Design review of the part built by this model. Coordinates are the model's own, in mm. Round coordinates to 2 decimals unless told otherwise and drop trailing zeros. Loops run counter-clockwise (first coordinate to the right, second up) from the corner with the lowest first, then second, coordinate; pieces in that order, holes last. Notation, with made-up numbers: (82, 11.25) - (88, 11.25) arc R22 ccw to (88, 30.25) - close; hole circle Ø11 at (-7, 57). An arc over 180 degrees is marked (long way). Return JSON: item names as keys, results as strings. Group by question number.
(1) We need section C-C, the plane x = -12.7. Write out the cut boundary in (y, z).
(2) We need section A-A, the plane y = -19.05. Write out the cut boundary in (x, z) (3 decimals).
(3) We need section B-B, the plane x = 0. Write out the cut boundary in (y, z), and give its area (3 significant figures).
(4) Wall thickness on L1, parallel to Y at x = -31.75, z = -7 (3 decimals); L2, parallel to Y at x = 0, z = -6; L3, parallel to Y at x = 12.7, z = -12: over which ranges is each line inside the solid? List them lowest first. Write a range as [from, to].
(5) The part is to be moulded in two halves that separate along Y. For faces 1 (the flat face through (-1, -25.4, -13)), 2 (the flat face through (-1, 6, -25.4)), 3 (the cylindrical face through (3.937, 1.24, -12.522)), 4 (the cylindrical face through (34.92, -18.91, -12.88)), say which applies: pulls with the +Y half, pulls with the -Y half, needs draft (parallel to the pull), parting line crosses it, or undercut.
(6) We need section D-D, the plane z = -22.25. Give the number of separate pieces and of enclosed holes in the cut face, and give its area (3 significant figures).
from build123d import *

# Parameters (mm, degrees)
SKETCH_1_W          = 76.2
SKETCH_1_H          = 50.8
EXTRUDE_1_DEPTH     = 25.4
SKETCH_2_R          = 4.1275
CUT_EXTRUDE_1_DEPTH = 25.4
SKETCH_3_R          = 3.175
CUT_EXTRUDE_2_DEPTH = 26.4
SKETCH_4_R          = 3.175
CUT_EXTRUDE_3_DEPTH = 25.4
SKETCH_5_R          = 4.7625
CUT_EXTRUDE_4_DEPTH = 25.4
SKETCH_6_R          = 4.7625
CUT_EXTRUDE_5_DEPTH = 25.4


with BuildPart() as part:
    # 草图1 → 凸台-拉伸1 (new body)
    with BuildSketch(Plane.XY):
        Rectangle(SKETCH_1_W, SKETCH_1_H)
    extrude(amount=-EXTRUDE_1_DEPTH)

    # 草图2 → 切除-拉伸1 (cut)
    with BuildSketch(Plane.XY):
        Circle(SKETCH_2_R)
    extrude(amount=-CUT_EXTRUDE_1_DEPTH, mode=Mode.SUBTRACT)

    # 草图3 → 切除-拉伸2 (cut, through all)
    with BuildSketch(Plane(origin=(0, 0, -25.4), x_dir=(-1, 0, 0), z_dir=(0, 0, -1))):
        with Locations((-31.75, 19.05)):
            Circle(SKETCH_3_R)
        with Locations((31.75, 19.05)):
            Circle(SKETCH_3_R)
    extrude(amount=-CUT_EXTRUDE_2_DEPTH, mode=Mode.SUBTRACT)

    # 草图4 → 切除-拉伸3 (cut)
    with BuildSketch(Plane(origin=(0, 0, -25.4), x_dir=(-1, 0, 0), z_dir=(0, 0, -1))):
        with Locations((-31.75, -19.05)):
            Circle(SKETCH_4_R)
        with Locations((31.75, -19.05)):
            Circle(SKETCH_4_R)
    extrude(amount=-CUT_EXTRUDE_3_DEPTH, mode=Mode.SUBTRACT)

    # 草图5 → 切除-拉伸4 (cut)
    with BuildSketch(Plane(origin=(0, 0, -25.4), x_dir=(-1, 0, 0), z_dir=(0, 0, -1))):
        with Locations((0, 12.7)):
            Circle(SKETCH_5_R)
        with Locations((0, -12.7)):
            Circle(SKETCH_5_R)
    extrude(amount=-CUT_EXTRUDE_4_DEPTH, mode=Mode.SUBTRACT)

    # 草图6 → 切除-拉伸5 (cut)
    with BuildSketch(Plane(origin=(0, 0, -25.4), x_dir=(-1, 0, 0), z_dir=(0, 0, -1))):
        with Locations((-12.7, 0)):
            Circle(SKETCH_6_R)
        with Locations((12.7, 0)):
            Circle(SKETCH_6_R)
    extrude(amount=-CUT_EXTRUDE_5_DEPTH, mode=Mode.SUBTRACT)


solid = part.part
Solutions:
{
 "1": {"outline": "(-25.4, -25.4) - (-4.76, -25.4) - (-4.76, 0) - (-25.4, 0) - close; (4.76, -25.4) - (25.4, -25.4) - (25.4, 0) - (4.76, 0) - close"},
 "2": {"outline": "(-38.1, -25.4) - (-34.925, -25.4) - (-34.925, 0) - (-38.1, 0) - close; (-28.575, -25.4) - (28.575, -25.4) - (28.575, 0) - (-28.575, 0) - close; (34.925, -25.4) - (38.1, -25.4) - (38.1, 0) - (34.925, 0) - close"},
 "3": {"outline": "(-25.4, -25.4) - (-17.46, -25.4) - (-17.46, 0) - (-25.4, 0) - close; (-7.94, -25.4) - (-4.13, -25.4) - (-4.13, 0) - (-7.94, 0) - close; (4.13, -25.4) - (7.94, -25.4) - (7.94, 0) - (4.13, 0) - close; (17.46, -25.4) - (25.4, -25.4) - (25.4, 0) - (17.46, 0) - close", "area": "597 mm^2"},
 "4": {"L1": "[-25.4, -22.225], [-15.875, 15.875], [22.225, 25.4]", "L2": "[-25.4, -17.46], [-7.94, -4.13], [4.13, 7.94], [17.46, 25.4]", "L3": "[-25.4, -4.76], [4.76, 25.4]"},
 "5": {"face 1": "pulls with the -Y half", "face 2": "needs draft", "face 3": "undercut", "face 4": "undercut"},
 "6": {"separate pieces": "1", "enclosed holes": "9", "area": "3,410 mm^2"}
}
